Check sheet for the modelled part. Datum: model origin and axes. Units: mm. Give positions to 0.01 mm unless a question says otherwise; leave off trailing zeros. Order: outer loops, then holes, each group sorted by start corner. A loop starts at its lowest first (then second) coordinate and runs counter-clockwise, first axis right, second up.
```python
from build123d import *

# Parameters (mm, degrees)
F0_W           = 92
F0_H           = 5
F1_DEPTH       = 35
F3_D           = 5.25
F3_DEPTH       = 5
F3_CBORE_D     = 9.75
F3_CBORE_DEPTH = 1.6
F3_TIP         = 1.5772591249
F4_D           = 2.5
F4_DEPTH       = 13.5
F4_TIP         = 0.7510757738
F2_W           = 5.4
F2_H           = 35
F5_DEPTH       = 5


with BuildPart() as f1:
    # F0 (on Front) → F1 (new body)
    with BuildSketch(Plane.XZ):
        with Locations((0, 2.5)):
            Rectangle(F0_W, F0_H)
    extrude(amount=F1_DEPTH)

    # F3
    with Locations(Plane.XY.offset(5)):
        with Locations((35.65, -20)):
            CounterBoreHole(F3_D / 2, F3_CBORE_D / 2, F3_CBORE_DEPTH, depth=F3_DEPTH)
            with Locations((0, 0, -(F3_DEPTH + F3_TIP / 2))):  # 118° drill point
                Cone(0, F3_D / 2, F3_TIP, mode=Mode.SUBTRACT)

    # F4
    with Locations(Plane.XY.offset(5)):
        with Locations((-38, -20.5), (-17, -20.5), (4, -20.5), (-17, -28.5)):
            Hole(F4_D / 2, depth=F4_DEPTH)
            with Locations((0, 0, -(F4_DEPTH + F4_TIP / 2))):  # 118° drill point
                Cone(0, F4_D / 2, F4_TIP, mode=Mode.SUBTRACT)

    # F2 (on face) → F5 (cut)
    with BuildSketch(Plane.XY.offset(5)):
        with Locations((43.3, -17.5)):
            Rectangle(F2_W, F2_H)
    extrude(amount=-F5_DEPTH, mode=Mode.SUBTRACT)


solid = f1.part
```
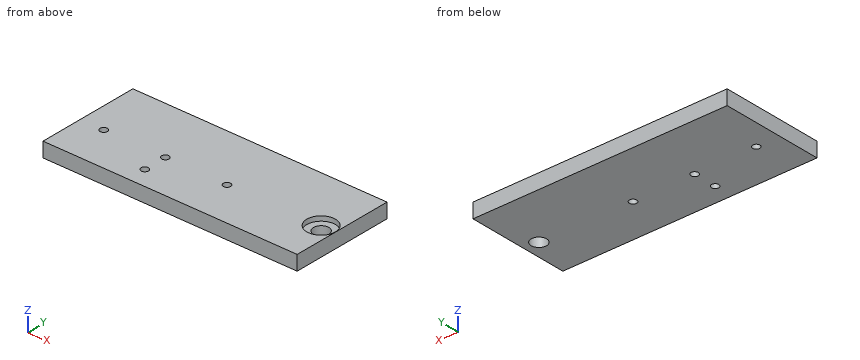
(1) Cross-section at A-A on y = -28.5. Enter the section's corners in (x, z).
Response values:
outline: (-46, 0) - (-18.25, 0) - (-18.25, 5) - (-46, 5) - close; (-15.75, 0) - (40.6, 0) - (40.6, 5) - (-15.75, 5) - close
(2) Material ranges on L1, parallel to Y at x = -17, z = 3.75; L2, parallel to Y at x = 4, z = 1; L3, parallel to Y at x = 35.65, z = 4.7 (3 decimals), recorded low to high.
Response values:
L1: y = -35 to -29.75, -27.25 to -21.75, -19.25 to 0
L2: y = -35 to -21.75, -19.25 to 0
L3: y = -35 to -24.875, -15.125 to 0
(3) Cross-section at C-C on x = 4. Enter the section's corners in (y, z), then the cut area to 4 significant figures.
Response values:
outline: (-35, 0) - (-21.75, 0) - (-21.75, 5) - (-35, 5) - close; (-19.25, 0) - (0, 0) - (0, 5) - (-19.25, 5) - close
area: 162.5 mm2
(4) Gauge pin test, flat end, axial feed: pin 1 Ø4 at (x, y) = (-17, -20.5) entering from +Z. Record the tip position at first contact, or that the pin passes through.
Response values:
pin 1: stops at z = 5
(5) Cross-section at B-B on x = 35.65. Enter the section's corners in (y, z) (3 decimals), then the cut area to 3 significant figures.
Response values:
outline: (-35, 0) - (-22.625, 0) - (-22.625, 3.4) - (-24.875, 3.4) - (-24.875, 5) - (-35, 5) - close; (-17.375, 0) - (0, 0) - (0, 5) - (-15.125, 5) - (-15.125, 3.4) - (-17.375, 3.4) - close
area: 142 mm2
